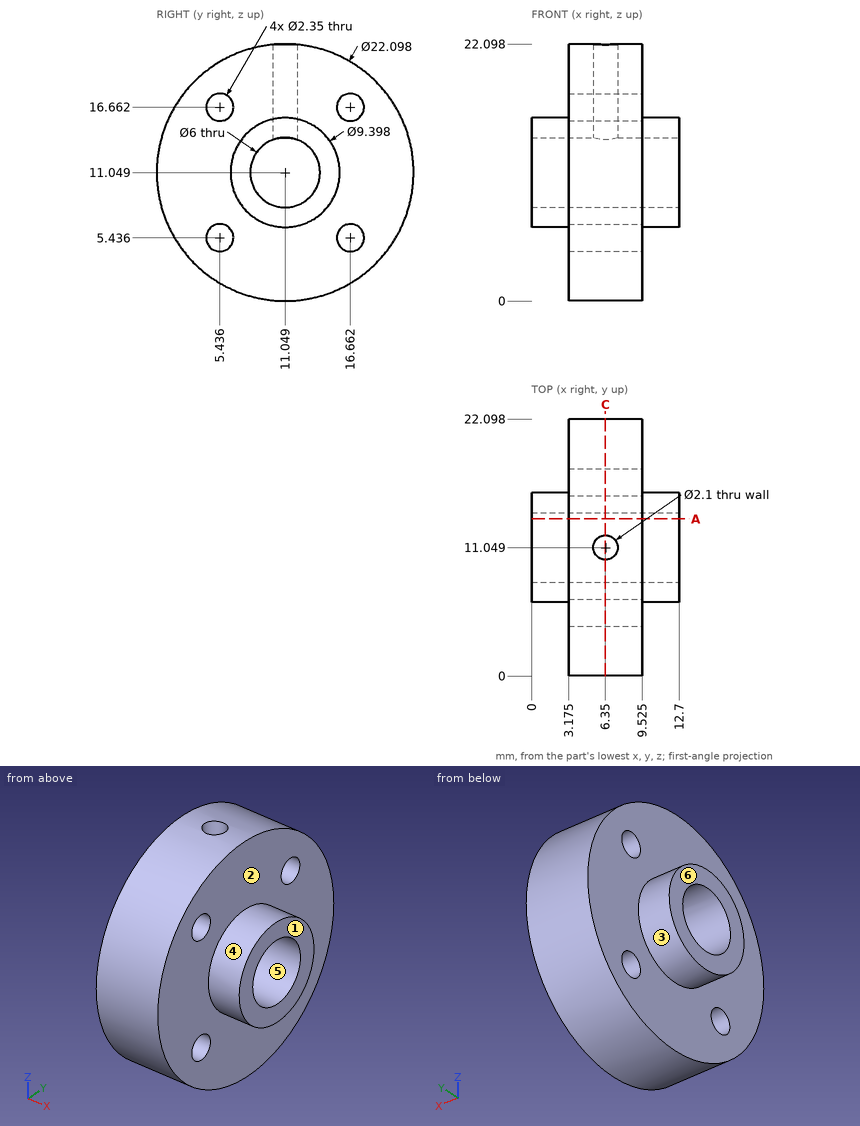
For this review, use the dimensioned drawing (mm, ordinates from the lowest corner) and the shaded views. A direction names the side the tool comes from. Round coordinates to 2 decimals unless told otherwise and drop trailing zeros. Order: outer loops, then holes, each group sorted by start corner. A loop starts at its lowest first (then second) coordinate and runs counter-clockwise, first axis right, second up. Notation, with made-up numbers: M 10.25,40 L 24.25,40 A24 cw 24.25,69 Z; hole C -12.5,-11.5 d7. An arc over 180 degrees is marked long. Write each question's results on one line, items separated by ' | '. Start each with the question number.
1. Draft analysis for pull direction Y (two halves, no side actions). For the marked faces 4, 5 and 6, state which applies: pulls with the +Y half, pulls with the -Y half, needs draft (parallel to the pull), parting line crosses it, or undercut.
2. Clearance check with flat-ended pins moving along their axes: pin 1 Ø8 at (y, z) = (17, 2.5) entering from +X (3 decimals); pin 2 Ø10 at (y, z) = (19.5, 8.5) entering from +X; pin 3 Ø4 at (y, z) = (5.44, 16.66) entering from -X (3 decimals); pin 4 Ø6 at (x, y) = (1.5, 14) entering from -Z. State where each tip first meets the part, or that it passes through.
3. Add section C-C (x = 6.35). State how many separate pieces and enclosed holes the cut face has, then the cut area to 3 significant figures.
4. Add section A-A (y = 13.5). State the section outline as (x, z) points (1 decimal).
5. Tool access review of the marked faces 1, 2 and 3: name each direction out of +Z, -Z, +X, -X, +Y, -Y from which nothing blocks a thin tool from reaching the whole face with its end or side.
6. To check wall thickness, follow L1, parallel to Y at x = 7.75, z = 17.25 (1 decimal); L2, parallel to X at y = 21, z = 9.5 (1 decimal). State the ranges of each line that lie inside material, in increasing order. Write a range as [from, to].
Output values:
1) face 4: parting line crosses it | face 5: undercut | face 6: needs draft
2) pin 1: x = 9.525 | pin 2: x = 12.7 | pin 3: x = 3.175 | pin 4: z = 0.01
3) separate pieces: 1 | enclosed holes: 4 | area: 321 mm^2
4) outline: M 0,7 L 3.2,7 L 3.2,0.3 L 9.5,0.3 L 9.5,7 L 12.7,7 L 12.7,9.3 L 0,9.3 Z; M 0,12.8 L 12.7,12.8 L 12.7,15.1 L 9.5,15.1 L 9.5,21.8 L 3.2,21.8 L 3.2,15.1 L 0,15.1 Z
5) face 1: +Z, -Z, +X, +Y, -Y | face 2: +X | face 3: -X
6) L1: [1.9, 4.4], [6.5, 15.6], [17.7, 20.2] | L2: [3.2, 9.5]
